Source: CAD feature listing. Evaluate the final solid. Frame: model axes, mm. Face numbers are marked on the shaded views. A direction names the side the tool comes from. Round coordinates to 2 decimals unless told otherwise and drop trailing zeros. Order: outer loops, then holes, each group sorted by start corner. A loop starts at its lowest first (then second) coordinate and runs counter-clockwise, first axis right, second up. Notation, with made-up numbers: M 5.25,29.5 L 47.25,29.5 A34 ccw 47.25,66.5 Z; hole C -7,-22 d5. An arc over 180 degrees is marked long. Answer as CSV lines item,"result". Start each with the question number.
Item 1: Section query D-D on z = -15.5. Return the cut outline in (x, y), plus the area to 3 significant figures.
Item 2: Section query A-A on z = -10. Return the cut outline in (x, y).
Item 3: Section query C-C on z = 10. Return the cut outline in (x, y), plus the area to 3 significant figures.
Item 4: Pull-direction query (X, two-part tool) for the marked faces 1, 2, 3 and 4; classes: +X half, -X half, draft (parallel to the pull), parting line (faces both ways), or undercut.
Item 5: Section query B-B on x = 0. Return the cut outline in (y, z), plus the area to 3 significant figures.
Item 6: Line query: line 1 (X direction, y = 19.75, z = 17.5); line 2 (X direction, y = 23.5, z = -20.5); line 3 (Z direction, x = -17.5, y = 13.25). Output: solid intervals per line, ascending. Write a range as [from, to].
Item 7: First-contact query: P1, Ø1.5, axis at x = 12.5, z = 11.5, coming from the +Y side; P2, Ø2, axis at x = -6, y = 5, coming from the -Z side; P3, Ø4.5, axis at x = -14.45, z = -4.75, coming from the +Y side. Flat tips, straight axial feed; report the tip coordinate or a pass-through.
Item 8: Set-up query: the marked faces 5 and 6. Return all of +Z, -Z, +X, -X, +Y, -Y with unobstructed straight access to the full face (end or side cutting, diameter ignored); none if empty.
from build123d import *

# Parameters (mm, degrees)
EXTRUDE_1_DEPTH     = 25
CUT_EXTRUDE_1_DEPTH = 10
SKETCH_5_W          = 41.777974616
SKETCH_5_H          = 18.894782553
EXTRUDE_4_DEPTH     = 7.1
SKETCH_7_R          = 1.75
CUT_EXTRUDE_2_DEPTH = 44.301270189
FILLET_1_R          = 3


with BuildPart() as part:
    # 草图1 → 凸台-拉伸1 (new body)
    with BuildSketch(Plane(origin=(0, 0, 0), x_dir=(1, 0, 0), z_dir=(0, 1, 0))):
        with BuildLine():
            Line((-25, -25), (25, -25))
            Line((25, -25), (25, 25))
            Line((25, 25), (12.530461135, 25))
            Line((12.530461135, 25), (12.530461135, -7.120248206))
            Line((12.530461135, -7.120248206), (15.530461135, -7.120248206))
            ThreePointArc((15.530461135, -7.120248206), (15.990080543, -7.310628798), (16.180461135, -7.770248206))
            Line((16.180461135, -7.770248206), (16.180461135, -8.120248206))
            Line((16.180461135, -8.120248206), (17.530461135, -8.120248206))
            ThreePointArc((17.530461135, -8.120248206), (17.990080543, -8.310628798), (18.180461135, -8.770248206))
            Line((18.180461135, -8.770248206), (18.180461135, -10.898803743))
            Line((18.180461135, -10.898803743), (19.204850948, -10.898803743))
            Line((19.204850948, -10.898803743), (19.204850948, -16.766546625))
            Line((19.204850948, -16.766546625), (18.180461135, -16.766546625))
            Line((18.180461135, -16.766546625), (18.180461135, -18.770248206))
            ThreePointArc((18.180461135, -18.770248206), (17.990080543, -19.229867614), (17.530461135, -19.420248206))
            Line((17.530461135, -19.420248206), (13.530461135, -19.420248206))
            ThreePointArc((13.530461135, -19.420248206), (13.282973762, -19.522760833), (13.180461135, -19.770248206))
            Line((13.180461135, -19.770248206), (13.180461135, -21.770248206))
            ThreePointArc((13.180461135, -21.770248206), (12.990080543, -22.229867614), (12.530461135, -22.420248206))
            Line((12.530461135, -22.420248206), (-12.469538865, -22.420248206))
            ThreePointArc((-12.469538865, -22.420248206), (-12.929158272, -22.229867614), (-13.119538865, -21.770248206))
            Line((-13.119538865, -21.770248206), (-13.119538865, -19.770248206))
            ThreePointArc((-13.119538865, -19.770248206), (-13.222051491, -19.522760833), (-13.469538865, -19.420248206))
            Line((-13.469538865, -19.420248206), (-17.469538865, -19.420248206))
            ThreePointArc((-17.469538865, -19.420248206), (-17.929158272, -19.229867614), (-18.119538865, -18.770248206))
            Line((-18.119538865, -18.770248206), (-18.119538865, -16.766546625))
            Line((-18.119538865, -16.766546625), (-18.180461135, -16.766546625))
            Line((-18.180461135, -16.766546625), (-19.204850948, -16.766546625))
            Line((-19.204850948, -16.766546625), (-19.204850948, -10.898803743))
            Line((-19.204850948, -10.898803743), (-18.180461135, -10.898803743))
            Line((-18.180461135, -10.898803743), (-18.119538865, -10.898803743))
            Line((-18.119538865, -10.898803743), (-18.119538865, -8.770248206))
            ThreePointArc((-18.119538865, -8.770248206), (-17.929158272, -8.310628798), (-17.469538865, -8.120248206))
            Line((-17.469538865, -8.120248206), (-16.119538865, -8.120248206))
            Line((-16.119538865, -8.120248206), (-16.119538865, -7.770248206))
            ThreePointArc((-16.119538865, -7.770248206), (-15.929158272, -7.310628798), (-15.469538865, -7.120248206))
            Line((-15.469538865, -7.120248206), (-14.200297417, -7.120248206))
            Line((-14.200297417, -7.120248206), (-14.200297417, 1.071122011))
            Line((-14.200297417, 1.071122011), (-11.261897063, 1.071122011))
            Line((-11.261897063, 1.071122011), (-11.261897063, 25))
            Line((-11.261897063, 25), (-25, 25))
            Line((-25, 25), (-25, -25))
        make_face()
    extrude(amount=EXTRUDE_1_DEPTH)

    # 草图2 → 切除-拉伸1 (cut)
    with BuildSketch(Plane.XY.offset(25)):
        with BuildLine():
            Line((7.139013901, 25), (-7.139013901, 25))
            ThreePointArc((-7.139013901, 25), (0, 17.860986099), (7.139013901, 25))
        make_face()
    extrude(amount=-CUT_EXTRUDE_1_DEPTH, mode=Mode.SUBTRACT)

    # 草图5 → 凸台-拉伸4 (add)
    with BuildSketch(Plane.XZ):
        with Locations((0, 13.870801672)):
            Rectangle(SKETCH_5_W, SKETCH_5_H)
    extrude(amount=-EXTRUDE_4_DEPTH)

    # 草图7 → 切除-拉伸2 (cut, through all)
    with BuildSketch(Plane(origin=(0, 25, 0), x_dir=(1, 0, 0), z_dir=(0, 1, 0))):
        with Locations(Location((15.550997874, 4.753034163, 0), (0, 0, 270))):
            Circle(SKETCH_7_R)
        with Locations(Location((15.550997874, 14.753034163, 0), (0, 0, 270))):
            Circle(SKETCH_7_R)
        with Locations(Location((-14.449002126, 4.753034163, 0), (0, 0, 270))):
            Circle(SKETCH_7_R)
        with Locations(Location((-14.449002126, 14.753034163, 0), (0, 0, 270))):
            Circle(SKETCH_7_R)
    extrude(amount=-CUT_EXTRUDE_2_DEPTH, mode=Mode.SUBTRACT)

    # 圆角1
    fillet_1_edges = [part.edges().sort_by_distance(p)[0] for p in [
        (-0.834918141, 0, 4.423410395),
        (0, 0, 25),
        (25, 12.5, -25),
        (25, 12.5, 25),
        (-25, 12.5, 25),
        (-25, 12.5, -25),
    ]]
    fillet(fillet_1_edges, radius=FILLET_1_R)


solid = part.part
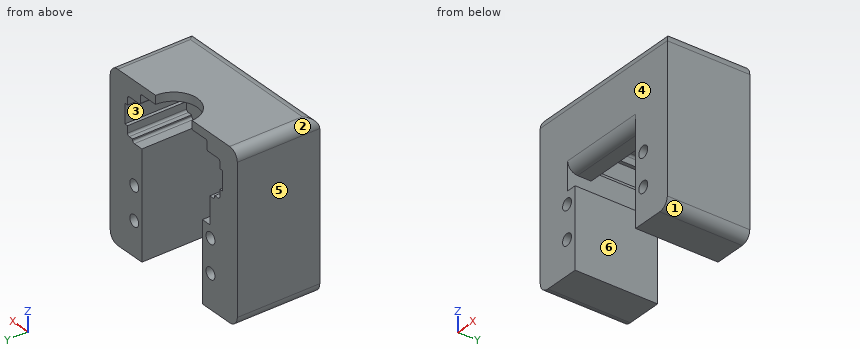
Results:
1,outline,"M -25,0 L -16.03,0 L -16.03,25 L -25,25 Z; M -12.87,0 L -11.26,0 L -11.26,25 L -12.87,25 Z; M 12.53,0 L 13.97,0 L 13.97,25 L 12.53,25 Z; M 17.13,0 L 25,0 L 25,25 L 17.13,25 Z"
1,area,"497 mm^2"
2,outline,"M -25,0 L -11.26,0 L -11.26,25 L -25,25 Z; M 12.53,0 L 25,0 L 25,25 L 12.53,25 Z"
3,outline,"M -25,0 L 25,0 L 25,25 L 18.18,25 L 18.18,7.1 L -18.12,7.1 L -18.12,25 L -25,25 Z"
3,area,"600 mm^2"
4,face 1,"+X half"
4,face 2,"-X half"
4,face 3,"undercut"
4,face 4,"draft"
5,outline,"M 0,7.42 A3 ccw 3,4.42 L 7.1,4.42 L 7.1,22.42 L 17.86,22.42 L 17.86,25 L 3,25 A3 ccw 0,22 Z"
5,area,"170 mm^2"
6,line 1,"[-25, -18.12], [18.18, 25]"
6,line 2,"[-25, -11.26], [12.53, 25]"
6,line 3,"[-25, 8.12], [19.42, 25]"
7,P1,"y = 7.1"
7,P2,"z = 4.42"
7,P3,"y = 25"
8,face 5,"+Z, -Z, -X, +Y, -Y"
8,face 6,"-Z, +Y, -Y"
